Verification items for the finished model (mm, model axes). A direction names the side the tool comes from. Coordinates: 2 decimals unless noted, no trailing zeros. Order: outer loops, then holes, each group sorted by start corner. A loop starts at its lowest first (then second) coordinate and runs counter-clockwise, first axis right, second up. Notation, with made-up numbers: (7.25, -31) - (47.25, -31) arc R14 cw to (47.25, -14) - close; hole circle Ø3 at (-35.75, 44). An arc over 180 degrees is marked (long way). Answer as CSV lines item,"result". Start each with the question number.
1. Section check C-C (x = -7.25). Record the cut outline in (y, z).
2. Section check B-B (z = 0). Record the cut outline in (x, y) (3 decimals).
3. Go/stop test with flat-tipped pins: pin 1 (5 mm diameter, centred on x = 0, z = 0, fed in from +Y); pin 2 (1 mm diameter, centred on x = -7.5, z = 7.5, fed in from -Y); pin 3 (1 mm diameter, centred on y = 1.5, z = -7, fed in from +X); pin 4 (4 mm diameter, centred on x = 2, z = -7, fed in from +Y). Record where each tip stops, or that it passes through.
4. Set-up check for faces 4 (the cylindrical face through (-8.116, 1.134, -2.885)), 5 (the cylindrical face through (-1.352, 3.828, -4.292)), 6 (the cylindrical face through (0.811, 0.394, -2.575)): record each of +Z, -Z, +X, -X, +Y, -Y from which the full face is reachable in a straight line by a thin tool's end or side.
5. Mould release check, pull along Z, two halves, no side actions. Record for faces 1 (the cylindrical face through (4.654, 1.134, -5.58)), 2 (the cylindrical face through (-9.76, 1.13, -2.17)), 3 (the flat face through (-2.1, 2.3, 4.3)): pulls with the +Z half, pulls with the -Z half, needs draft (parallel to the pull), parting line crosses it, or undercut.
6. Material ranges on L1, parallel to X at y = 0.7, z = 1.25; L2, parallel to Z at x = -7, y = 1.1; L3, parallel to X at y = 1.3, z = -2.5, recorded low to high. Write a range as [from, to].
7. Section check A-A (x = 0). Record the cut outline in (y, z) (3 decimals), and give its area (3 significant figures).
8. Section check D-D (y = 4.35). Record the cut outline in (x, z).
from build123d import *

# Parameters (mm, degrees)
SKETCH1_R           = 10
SKETCH1_R_2         = 0.66
SKETCH1_R_3         = 1.5
BOSS_EXTRUDE1_DEPTH = 2.3
SKETCH2_R           = 4.5
SKETCH2_R_2         = 1.5
BOSS_EXTRUDE2_DEPTH = 3.1
SKETCH3_R           = 2.25
CUT_EXTRUDE1_DEPTH  = 3.6
SKETCH_1_R          = 0.66
CUT_EXTRUDE_1_DEPTH = 16.138031576
SKETCH_2_R          = 4.375
SKETCH_2_R_2        = 3.2
SKETCH_2_R_3        = 2.7
SKETCH_2_R_4        = 1.5
CUT_EXTRUDE_2_DEPTH = 0.8


with BuildPart() as part:
    # Sketch1 → Boss-Extrude1 (new body)
    with BuildSketch(Plane(origin=(0, 0, 0), x_dir=(1, 0, 0), z_dir=(0, 1, 0))):
        with Locations(Location((0, 0, 0), (0, 0, 270))):
            Circle(SKETCH1_R)
        with Locations(Location((-5.055813485, 5.055813485, 0), (0, 0, 270))):
            Circle(SKETCH1_R_2, mode=Mode.SUBTRACT)
        with Locations(Location((5.055813485, 5.055813485, 0), (0, 0, 270))):
            Circle(SKETCH1_R_2, mode=Mode.SUBTRACT)
        with Locations(Location((5.055813485, -5.055813485, 0), (0, 0, 270))):
            Circle(SKETCH1_R_2, mode=Mode.SUBTRACT)
        with Locations(Location((-5.055813485, -5.055813485, 0), (0, 0, 270))):
            Circle(SKETCH1_R_2, mode=Mode.SUBTRACT)
        with Locations(Location((0, 0, 0), (0, 0, 270))):
            Circle(SKETCH1_R_3, mode=Mode.SUBTRACT)
    extrude(amount=BOSS_EXTRUDE1_DEPTH)

    # Sketch2 → Boss-Extrude2 (add)
    with BuildSketch(Plane(origin=(0, 2.3, 0), x_dir=(1, 0, 0), z_dir=(0, 1, 0))):
        with Locations(Location((0, 0, 0), (0, 0, 90))):
            Circle(SKETCH2_R)
        with Locations(Location((0, 0, 0), (0, 0, 270))):
            Circle(SKETCH2_R_2, mode=Mode.SUBTRACT)
    extrude(amount=BOSS_EXTRUDE2_DEPTH)

    # Sketch3 → Cut-Extrude1 (cut)
    with BuildSketch(Plane(origin=(0, 5.4, 0), x_dir=(1, 0, 0), z_dir=(0, 1, 0))):
        with Locations(Location((0, 0, 0), (0, 0, 270))):
            Circle(SKETCH3_R)
    extrude(amount=-CUT_EXTRUDE1_DEPTH, mode=Mode.SUBTRACT)

    # ｽｹｯﾁ1 → ｶｯﾄ - 押し出し1 (cut, through all)
    with BuildSketch(Plane(origin=(0, 0, 0), x_dir=(-1, 0, 0), z_dir=(0, -1, 0))):
        with Locations(Location((-2.580939751, -7.53068722, 0), (0, 0, 90))):
            Circle(SKETCH_1_R)
        with Locations(Location((-7.53068722, -2.580939751, 0), (0, 0, 90))):
            Circle(SKETCH_1_R)
        with Locations(Location((-7.53068722, 2.580939751, 0), (0, 0, 90))):
            Circle(SKETCH_1_R)
        with Locations(Location((-2.580939751, 7.53068722, 0), (0, 0, 90))):
            Circle(SKETCH_1_R)
        with Locations(Location((2.580939751, 7.53068722, 0), (0, 0, 90))):
            Circle(SKETCH_1_R)
        with Locations(Location((7.53068722, 2.580939751, 0), (0, 0, 90))):
            Circle(SKETCH_1_R)
        with Locations(Location((7.53068722, -2.580939751, 0), (0, 0, 90))):
            Circle(SKETCH_1_R)
        with Locations(Location((2.580939751, -7.53068722, 0), (0, 0, 90))):
            Circle(SKETCH_1_R)
    extrude(amount=-CUT_EXTRUDE_1_DEPTH, mode=Mode.SUBTRACT)

    # ｽｹｯﾁ2 → ｶｯﾄ - 押し出し2 (cut)
    # profile 1 of 2: a face of its own
    with BuildSketch(Plane(origin=(0, 0, 0), x_dir=(-1, 0, 0), z_dir=(0, -1, 0))):
        with Locations(Location((0, 0, 0), (0, 0, 90))):
            Circle(SKETCH_2_R)
        with Locations(Location((0, 0, 0), (0, 0, 90))):
            Circle(SKETCH_2_R_2, mode=Mode.SUBTRACT)
    # profile 2 of 2: a face of its own
    with BuildSketch(Plane(origin=(0, 0, 0), x_dir=(-1, 0, 0), z_dir=(0, -1, 0))):
        with Locations(Location((0, 0, 0), (0, 0, 90))):
            Circle(SKETCH_2_R_3)
        with Locations(Location((0, 0, 0), (0, 0, 90))):
            Circle(SKETCH_2_R_4, mode=Mode.SUBTRACT)
    extrude(amount=-CUT_EXTRUDE_2_DEPTH, mode=Mode.SUBTRACT)


solid = part.part
Evaluation:
1,outline,"(0, -6.89) - (2.3, -6.89) - (2.3, -3.18) - (0, -3.18) - close; (0, -1.98) - (2.3, -1.98) - (2.3, 1.98) - (0, 1.98) - close; (0, 3.18) - (2.3, 3.18) - (2.3, 6.89) - (0, 6.89) - close"
2,outline,"(-10, 0) - (-4.375, 0) - (-4.375, 0.8) - (-3.2, 0.8) - (-3.2, 0) - (-2.7, 0) - (-2.7, 0.8) - (-1.5, 0.8) - (-1.5, 1.8) - (-2.25, 1.8) - (-2.25, 5.4) - (-4.5, 5.4) - (-4.5, 2.3) - (-10, 2.3) - close; (1.5, 0.8) - (2.7, 0.8) - (2.7, 0) - (3.2, 0) - (3.2, 0.8) - (4.375, 0.8) - (4.375, 0) - (10, 0) - (10, 2.3) - (4.5, 2.3) - (4.5, 5.4) - (2.25, 5.4) - (2.25, 1.8) - (1.5, 1.8) - close"
3,pin 1,"stops at y = 5.4"
3,pin 2,"passes through"
3,pin 3,"stops at x = 7.6"
3,pin 4,"stops at y = 2.3"
4,face 4,"+Y, -Y"
4,face 5,"+Y"
4,face 6,"-Y"
5,face 1,"undercut"
5,face 2,"parting line crosses it"
5,face 3,"needs draft"
6,L1,"x = [-9.92, -4.19], [-2.95, -2.39], [2.39, 2.95], [4.19, 9.92]"
6,L2,"z = [-7.14, -2.97], [-2.19, 2.19], [2.97, 7.14]"
6,L3,"x = [-9.68, -8.19], [-6.88, 6.88], [8.19, 9.68]"
7,outline,"(0, -10) - (2.3, -10) - (2.3, -4.5) - (5.4, -4.5) - (5.4, -2.25) - (1.8, -2.25) - (1.8, -1.5) - (0.8, -1.5) - (0.8, -2.7) - (0, -2.7) - (0, -3.2) - (0.8, -3.2) - (0.8, -4.375) - (0, -4.375) - close; (0, 2.7) - (0.8, 2.7) - (0.8, 1.5) - (1.8, 1.5) - (1.8, 2.25) - (5.4, 2.25) - (5.4, 4.5) - (2.3, 4.5) - (2.3, 10) - (0, 10) - (0, 4.375) - (0.8, 4.375) - (0.8, 3.2) - (0, 3.2) - close"
7,area,"48.5 mm²"
8,outline,"circle Ø9 at (0, 0); hole circle Ø4.5 at (0, 0)"
